Source: CAD feature listing. Evaluate the final solid. Frame: model axes, mm. Face numbers are marked on the shaded views. A direction names the side the tool comes from. Coordinates: 2 decimals unless noted, no trailing zeros. Write each loop counter-clockwise with the first axis right and the second up, starting at its lowest first coordinate (ties: lowest second). Pieces come first, ordered by that corner, then holes. Notation, with made-up numbers: (35, 43) -> (57, 43) arc R33 ccw to (57, 74) -> close; hole circle Ø4 at (88, 77.5). An arc over 180 degrees is marked (long way). One line per item, written item: value. Start each with the question number.
1. Mould query, pull axis X, two halves, no side actions, for the marked faces 1, 2 and 3. Classes: released by +X, released by -X, zero draft, split by the parting line, or undercut.
2. Section query D-D, the plane x = 2.25. Output: boundary loops of the cut face in (y, z), and give its area (3 significant figures).
3. Section query C-C, the plane z = 7.75. Output: boundary loops of the cut face in (x, y).
4. Section query A-A, the plane x = 0. Output: boundary loops of the cut face in (y, z).
5. Section query B-B, the plane y = -5.75. Output: boundary loops of the cut face in (x, z).
6. First-contact query: P1, Ø2.5, axis at x = 0, z = -9, coming from the -Y side; P2, Ø8, axis at y = 3, z = -9.5, coming from the -X side; P3, Ø7.5, axis at y = 2, z = 1, coming from the +X side. Flat tips, straight axial feed; report the tip coordinate or a pass-through.
7. Line query: line 1 (Z direction, x = 1.75, y = 3.5); line 2 (Y direction, x = 0, z = 2); line 3 (X direction, y = 3.95, z = 7). Output: solid intervals per line, ascending.
8. Access query for the marked faces 4, 5 and 6. Directions: +Z, -Z, +X, -X, +Y, -Y. A direction counts if a zero-diameter tool reaches every point of the face in a straight line with its end or side. Return the directions, or none.
Autodesk Inventor part; units mm, degrees
ref_plane "YZ Plane" through (0, 0, 0) normal (1, 0, 0) x (0, 1, 0)
ref_plane "XZ Plane" through (0, 0, 0) normal (0, 1, 0) x (-1, 0, 0)
ref_plane "XY Plane" through (0, 0, 0) normal (0, 0, 1) x (1, 0, 0)
sketch "Sketch1" plane through (0, 0, 0) normal (0, 1, 0) x (-1, 0, 0)
  circle A0 centre (0, 7) radius 2
  circle A1 centre (0, -7) radius 2
  line L0 (0, 7) -> (0, -7)
  line L1 (5, -12) -> (-5, -12)
  line L2 (-5, -12) -> (-5, 12)
  line L3 (-5, 12) -> (5, 12)
  line L4 (5, 12) -> (5, -12)
  point P0 (0, 0)
  point P1 (0, 0)
  point P2 (-5, 0)
  point P3 (0, -12)
  dimension "d0" = 4
  dimension "d1" = 4
  dimension "d2" = 14
  dimension "d3" = 10
  dimension "d4" = 24
extrude "Extrusion1" add sketch "Sketch1" along normal blind 5
sketch "Sketch2" plane through (5, 0, -12) normal (0, 0, -1) x (-1, 0, 0)
  circle A0 centre (5, -5) radius 6
  circle A1 centre (5, -5) radius 3
  line L0 (0, 0) -> (0, 5)
  line L1 (10, 0) -> (0, 0)
  line L2 (0, 0) -> (0, -1.6834)
  line L3 (10, 0) -> (10, -1.6834)
  line L4 (2, -10.1962) -> (8, -10.1962)
  point P0 (5, 0)
  dimension "d7" = 6
  dimension "d8" = 5
  dimension "d9" = 5
  dimension "d10" = 12
  dimension "d11" = 6
extrude "Extrusion2" add sketch "Sketch2" against normal blind 24 contours A0 L4 L1 | A0 L1 L3 | A0 L2 L1
sketch "Sketch3" plane through (-3, -10.1962, -12) normal (0, -1, 0) x (1, 0, 0)
  circle A0 centre (3, 3) radius 1.5
  line L0 (3, 3) -> (3, 12) construction
  dimension "d14" = 3
  dimension "d15" = 9
extrude "Extrusion3" cut sketch "Sketch3" against normal blind 6.25
properties part number "Metal_Bushing"
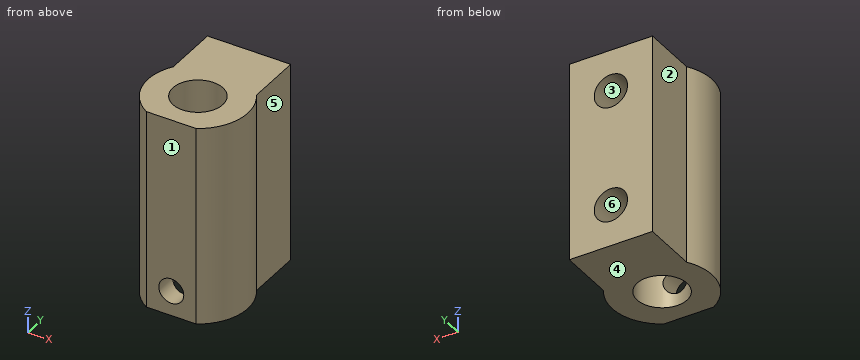
Computed values:
1. face 1: zero draft
1. face 2: released by -X
1. face 3: undercut
2. outline: (-10.2, -12) -> (-6.98, -12) -> (-6.98, 12) -> (-10.2, 12) -> close; (-3.02, -12) -> (5, -12) -> (5, 12) -> (-3.02, 12) -> close
2. area: 269 mm²
3. outline: (-5, -1.68) arc R6 ccw to (-3, -10.2) -> (3, -10.2) arc R6 ccw to (5, -1.68) -> (5, 5) -> (1.85, 5) -> (1.85, 0) -> (-1.85, 0) -> (-1.85, 5) -> (-5, 5) -> close; hole circle Ø6 at (0, -5)
4. outline: (-10.2, -12) -> (-8, -12) -> (-8, -10.5) -> (-10.2, -10.5) -> close; (-10.2, -7.5) -> (-8, -7.5) -> (-8, 12) -> (-10.2, 12) -> close; (-2, -12) -> (5, -12) -> (5, -9) -> (0, -9) -> (0, -5) -> (5, -5) -> (5, 5) -> (0, 5) -> (0, 9) -> (5, 9) -> (5, 12) -> (-2, 12) -> close
5. outline: (-5.95, -12) -> (-2.9, -12) -> (-2.9, 12) -> (-5.95, 12) -> close; (2.9, -12) -> (5.95, -12) -> (5.95, 12) -> (2.9, 12) -> close
6. P1: stops at y = -2.27
6. P2: stops at x = -5
6. P3: stops at x = 5.04
7. line 1: z = -12 to -7.97, -6.03 to 6.03, 7.97 to 12
7. line 2: y = -10.2 to -8, -2 to 5
7. line 3: x = -5 to -2, 2 to 5
8. face 4: -Z, +X, -X, +Y, -Y
8. face 5: +Z, -Z, +X, +Y
8. face 6: +Y
